Verification items for the finished model (mm, model axes). Face numbers are marked on the shaded views. Round coordinates to 2 decimals unless told otherwise and drop trailing zeros. Write each loop counter-clockwise with the first axis right and the second up, starting at its lowest first coordinate (ties: lowest second). Pieces come first, ordered by that corner, then holes. Notation, with made-up numbers: (-10, 32.5) - (49, 32.5) arc R14 ccw to (49, 49.5) - close; hole circle Ø3 at (28.25, 20.25). An arc over 180 degrees is marked (long way). Answer as a JSON object with one key per item and string values.
```python
from build123d import *

# Parameters (mm, degrees)
SKETCH1_W           = 50
SKETCH1_H           = 35
SKETCH1_R           = 5
SKETCH1_R_2         = 1.75
BOSS_EXTRUDE1_DEPTH = 5
FILLET1_R           = 10
FILLET2_R           = 2
SKETCH2_W           = 10
SKETCH2_H           = 6
BOSS_EXTRUDE2_DEPTH = 10
CHAMFER1_SIZE2      = 7.002075382
CHAMFER1_SIZE       = 10
SKETCH3_R           = 1
CUT_EXTRUDE1_DEPTH  = 62.846584384


with BuildPart() as part:
    # Sketch1 → Boss-Extrude1 (new body)
    with BuildSketch(Plane(origin=(0, 0, 0), x_dir=(1, 0, 0), z_dir=(0, 1, 0))):
        with Locations((25, 17.5)):
            Rectangle(SKETCH1_W, SKETCH1_H)
        with Locations(Location((22, 17.5, 0), (0, 0, 270))):
            Circle(SKETCH1_R, mode=Mode.SUBTRACT)
        with Locations(Location((47.5, 32, 0), (0, 0, 270))):
            Circle(SKETCH1_R_2, mode=Mode.SUBTRACT)
        with Locations(Location((47.5, 22, 0), (0, 0, 270))):
            Circle(SKETCH1_R_2, mode=Mode.SUBTRACT)
        with Locations(Location((47.5, 13, 0), (0, 0, 270))):
            Circle(SKETCH1_R_2, mode=Mode.SUBTRACT)
        with Locations(Location((47.5, 3, 0), (0, 0, 270))):
            Circle(SKETCH1_R_2, mode=Mode.SUBTRACT)
    extrude(amount=BOSS_EXTRUDE1_DEPTH)

    # Fillet1
    fillet1_edges = [part.edges().sort_by_distance(p)[0] for p in [
        (0, 2.5, 0),
        (0, 2.5, -35),
    ]]
    fillet(fillet1_edges, radius=FILLET1_R)

    # Fillet2
    fillet2_edges = [part.edges().sort_by_distance(p)[0] for p in [
        (50, 2.5, -35),
        (50, 2.5, 0),
    ]]
    fillet(fillet2_edges, radius=FILLET2_R)

    # Sketch2 → Boss-Extrude2 (add)
    with BuildSketch(Plane(origin=(0, 5, 0), x_dir=(1, 0, 0), z_dir=(0, 1, 0))):
        with Locations((39.8, 17.5)):
            Rectangle(SKETCH2_W, SKETCH2_H)
    extrude(amount=BOSS_EXTRUDE2_DEPTH)

    # Chamfer1
    chamfer1_edges = [part.edges().sort_by_distance(p)[0] for p in [
        (34.8, 15, -17.5),
    ]]
    chamfer1_side = [part.faces().sort_by_distance(p)[0] for p in [
        (34.8, 14.859958492, -17.5),
    ]]
    chamfer(chamfer1_edges, length=CHAMFER1_SIZE - 0.0001, length2=CHAMFER1_SIZE2 - 0.0001, reference=chamfer1_side[0])  # a hair under: the kernel refuses the full size

    # Sketch3 → Cut-Extrude1 (cut, through all)
    with BuildSketch(Plane(origin=(0, 5, 0), x_dir=(1, 0, 0), z_dir=(0, 1, 0))):
        with Locations(Location((5.7, 17.5, 0), (0, 0, 270))):
            Circle(SKETCH3_R)
        with Locations(Location((29.3, 17.5, 0), (0, 0, 270))):
            Circle(SKETCH3_R)
    extrude(amount=-CUT_EXTRUDE1_DEPTH, mode=Mode.SUBTRACT)


solid = part.part
```
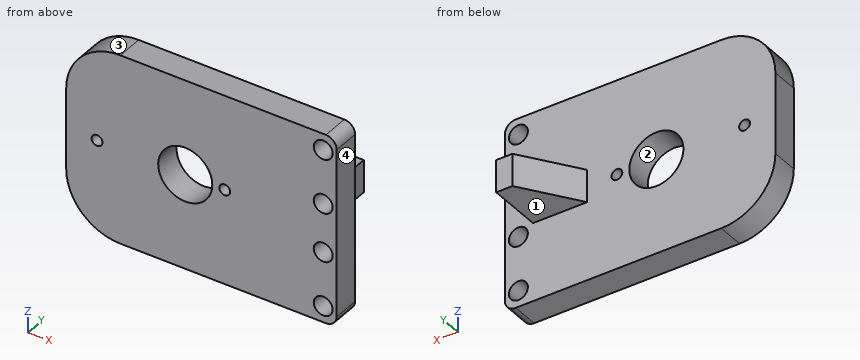
1. Cross-section at A-A (x = 29.3). Record the boundary of the cut face in (y, z), plus the area to 3 significant figures.
Completed:
{"outline": "(0, -35) - (5, -35) - (5, -18.5) - (0, -18.5) - close; (0, -16.5) - (5, -16.5) - (5, 0) - (0, 0) - close", "area": "165 mm^2"}
2. Cross-section at B-B (y = 2.25). Record the boundary of the cut face in (x, z).
Completed:
{"outline": "(0, -25) arc R10 ccw to (10, -35) - (48, -35) arc R2 ccw to (50, -33) - (50, -2) arc R2 ccw to (48, 0) - (10, 0) arc R10 ccw to (0, -10) - close; hole circle Ø2 at (5.7, -17.5); hole circle Ø10 at (22, -17.5); hole circle Ø2 at (29.3, -17.5); hole circle Ø3.5 at (47.5, -32); hole circle Ø3.5 at (47.5, -22); hole circle Ø3.5 at (47.5, -13); hole circle Ø3.5 at (47.5, -3)"}
3. Cross-section at D-D (z = -32). Record the boundary of the cut face in (x, y), plus the area to 3 significant figures.
Completed:
{"outline": "(2.86, 0) - (45.75, 0) - (45.75, 5) - (2.86, 5) - close; (49.25, 0) - (50, 0) - (50, 5) - (49.25, 5) - close", "area": "218 mm^2"}
4. Mould release check, pull along X, two halves, no side actions. Record for the marked faces 1, 2, 3 and 4: released by +X, released by -X, zero draft, split by the parting line, or undercut.
Completed:
{"face 1": "zero draft", "face 2": "undercut", "face 3": "released by -X", "face 4": "released by +X"}
5. Material ranges on probe 1 along X at (y, z) = (2.25, -13); probe 2 along Y at (x, z) = (33, -3); probe 3 along X at (y, z) = (4, -1.5), recorded low to high. Write a range as from..to.
Completed:
{"probe 1": "x = 0..19.82, 24.18..45.75, 49.25..50", "probe 2": "y = 0..5", "probe 3": "x = 4.73..46.6, 48.4..49.94"}
6. Cross-section at C-C (x = 46.5). Record the boundary of the cut face in (y, z).
Completed:
{"outline": "(0, -35) - (5, -35) - (5, -33.44) - (0, -33.44) - close; (0, -30.56) - (5, -30.56) - (5, -23.44) - (0, -23.44) - close; (0, -20.56) - (5, -20.56) - (5, -14.44) - (0, -14.44) - close; (0, -11.56) - (5, -11.56) - (5, -4.44) - (0, -4.44) - close; (0, -1.56) - (5, -1.56) - (5, 0) - (0, 0) - close"}
7. Go/stop test with flat-tipped pins: pin 1 (4.5 mm diameter, centred on x = 47.5, z = -13, fed in from +Y); pin 2 (1.8 mm diameter, centred on x = 5.7, z = -17.5, fed in from +Y); pin 3 (5 mm diameter, centred on x = 38.5, y = 8, fed in from +Z); pin 4 (6.5 mm diameter, centred on y = 9, z = -18.5, fed in from +X). Record where each tip stops, or that it passes through.
Completed:
{"pin 1": "stops at y = 5", "pin 2": "passes through", "pin 3": "stops at z = -14.5", "pin 4": "stops at x = 44.8"}
